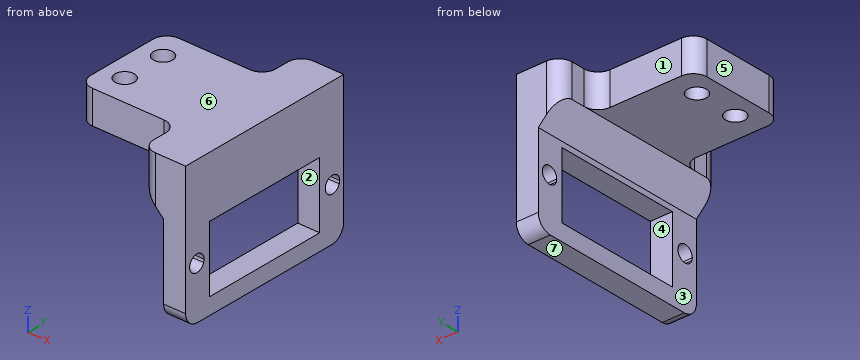
```python
from build123d import *

# Parameters (mm, degrees)
F0_W      = 4
F0_H      = 18
F1_DEPTH  = 26
F0_W_2    = 7
F2_DEPTH  = 6
F3_W      = 4
F3_H      = 18
F4_DEPTH  = 15
F5_W      = 4
F5_H      = 18
F6_DEPTH  = 15
F7_W      = 11.5
F7_H      = 5.5
F7_H_2    = 6
F7_H_3    = 0.5
F8_DEPTH  = 25
F9_DEPTH  = 15
F10_DEPTH = 18
F11_DEPTH = 2
F12_DEPTH = 6
F13_DEPTH = 6
F14_DEPTH = 11
F15_W     = 9
F15_H     = 8
F16_DEPTH = 30
F18_D     = 3.5
F19_W     = 18
F19_H     = 6
F20_DEPTH = 9
F21_W     = 18
F21_H     = 6
F22_DEPTH = 9
F23_SIZE  = 4
F24_DEPTH = 1.5
F25_DEPTH = 1.5
F26_R     = 2.5


with BuildPart() as f1:
    # F0 (on Top) → F1 (new body)
    with BuildSketch(Plane.XY):
        with Locations((9, 9)):
            Rectangle(F0_W, F0_H)
    extrude(amount=-F1_DEPTH)

    # F0 (on Top) → F2 (join)
    with BuildSketch(Plane.XY):
        with Locations((3.5, 9)):
            Rectangle(F0_W_2, F0_H)
        with Locations((9, 9)):
            Rectangle(F0_W, F0_H)
    extrude(amount=-F2_DEPTH)

    # F3 (on face) → F4 (join)
    with BuildSketch(Plane.XZ):
        with Locations((9, -17)):
            Rectangle(F3_W, F3_H)
    extrude(amount=F4_DEPTH)

    # F5 (on face) → F6 (join)
    with BuildSketch(Plane(origin=(0, 18, 0), x_dir=(-1, 0, 0), z_dir=(0, 1, 0))):
        with Locations((-9, -17)):
            Rectangle(F5_W, F5_H)
    extrude(amount=F6_DEPTH)

    # F7 (on face) → F8 (cut)
    with BuildSketch(Plane.YZ.offset(11)):
        with Locations((3.25, -13.75)):
            Rectangle(F7_W, F7_H)
        with Locations((14.75, -13.75)):
            Rectangle(F7_W, F7_H)
        with BuildLine():
            Line((24.5675133947, -17), (21.7390862699, -17))
            ThreePointArc((21.7390862699, -17), (23.1532998323, -18), (24.5675133947, -17))
        make_face()
        with BuildLine():
            Line((24.6532998323, -16.5), (21.6532998323, -16.5))
            ThreePointArc((21.6532998323, -16.5), (21.6749019928, -16.7536529681), (21.7390862699, -17))
            Line((21.7390862699, -17), (24.5675133947, -17))
            ThreePointArc((24.5675133947, -17), (24.6316976718, -16.7536529681), (24.6532998323, -16.5))
        make_face()
        with BuildLine():
            ThreePointArc((24.6532998323, -16.5), (23.1532998323, -15), (21.6532998323, -16.5))
            Line((21.6532998323, -16.5), (24.6532998323, -16.5))
        make_face()
        with Locations((14.75, -20)):
            Rectangle(F7_W, F7_H_2)
        with Locations((14.75, -16.75)):
            Rectangle(F7_W, F7_H_3)
        with Locations((3.25, -20)):
            Rectangle(F7_W, F7_H_2)
        with Locations((3.25, -16.75)):
            Rectangle(F7_W, F7_H_3)
        with BuildLine():
            ThreePointArc((-3.6532998323, -16.5), (-5.1532998323, -15), (-6.6532998323, -16.5))
            Line((-6.6532998323, -16.5), (-3.6532998323, -16.5))
        make_face()
        with BuildLine():
            Line((-3.6532998323, -16.5), (-6.6532998323, -16.5))
            ThreePointArc((-6.6532998323, -16.5), (-6.6316976718, -16.7536529681), (-6.5675133947, -17))
            Line((-6.5675133947, -17), (-3.7390862699, -17))
            ThreePointArc((-3.7390862699, -17), (-3.6749019928, -16.7536529681), (-3.6532998323, -16.5))
        make_face()
        with BuildLine():
            Line((-3.7390862699, -17), (-6.5675133947, -17))
            ThreePointArc((-6.5675133947, -17), (-5.1532998323, -18), (-3.7390862699, -17))
        make_face()
    extrude(amount=-F8_DEPTH, mode=Mode.SUBTRACT)

    # F9 (add): a face of the model
    f9_faces = [f1.faces().sort_by_distance(p)[0] for p in [
        (0, 9, -3),
    ]]
    extrude(f9_faces, amount=F9_DEPTH)

    # F10 (add): a face of the model
    f10_faces = [f1.faces().sort_by_distance(p)[0] for p in [
        (-1.4634146341, 0, -3.1951219512),
    ]]
    extrude(f10_faces, amount=F10_DEPTH)

    # F11 (cut): a face of the model
    f11_faces = [f1.faces().sort_by_distance(p)[0] for p in [
        (-1.4634146341, 18, -3.1951219512),
    ]]
    extrude(f11_faces, amount=-F11_DEPTH, mode=Mode.SUBTRACT)

    # F12 (cut): a face of the model
    f12_faces = [f1.faces().sort_by_distance(p)[0] for p in [
        (9, -15, -17),
    ]]
    extrude(f12_faces, amount=-F12_DEPTH, mode=Mode.SUBTRACT)

    # F13 (cut): a face of the model
    f13_faces = [f1.faces().sort_by_distance(p)[0] for p in [
        (9, 33, -17),
    ]]
    extrude(f13_faces, amount=-F13_DEPTH, mode=Mode.SUBTRACT)

    # F14 (add): a face of the model
    f14_faces = [f1.faces().sort_by_distance(p)[0] for p in [
        (-1.4634146341, 16, -3.1951219512),
    ]]
    extrude(f14_faces, amount=F14_DEPTH)

    # F15 (on face) → F16 (cut)
    with BuildSketch(Plane.YZ.offset(11)):
        with Locations((-13.5, -4)):
            Rectangle(F15_W, F15_H)
    extrude(amount=-F16_DEPTH, mode=Mode.SUBTRACT)

    # F18 (through all)
    with Locations(Plane.XY):
        with Locations((-11, 13), (-11, 5)):
            Hole(F18_D / 2)

    # F19 (on face) → F20 (cut)
    with BuildSketch(Plane.XZ.offset(9)):
        with Locations((-6, -3)):
            Rectangle(F19_W, F19_H)
    extrude(amount=-F20_DEPTH, mode=Mode.SUBTRACT)

    # F21 (on face) → F22 (cut)
    with BuildSketch(Plane(origin=(0, 27, 0), x_dir=(-1, 0, 0), z_dir=(0, 1, 0))):
        with Locations((6, -3)):
            Rectangle(F21_W, F21_H)
    extrude(amount=-F22_DEPTH, mode=Mode.SUBTRACT)

    # F23
    f23_edges = [f1.edges().sort_by_distance(p)[0] for p in [
        (7, 9, -6),
    ]]
    chamfer(f23_edges, length=F23_SIZE)

    # F24 (cut): a face of the model
    f24_faces = [f1.faces().sort_by_distance(p)[0] for p in [
        (8.0980392157, -9, -10.9019607843),
    ]]
    extrude(f24_faces, amount=-F24_DEPTH, mode=Mode.SUBTRACT)

    # F25 (cut): a face of the model
    f25_faces = [f1.faces().sort_by_distance(p)[0] for p in [
        (8.0980392157, 27, -10.9019607843),
    ]]
    extrude(f25_faces, amount=-F25_DEPTH, mode=Mode.SUBTRACT)

    # F26
    f26_edges = [f1.edges().sort_by_distance(p)[0] for p in [
        (9, 25.5, -26),
        (3, 25.5, -3),
        (-15, 18, -3),
        (9, -7.5, -26),
        (3, -7.5, -3),
        (3, 0, -3),
        (3, 18, -3),
        (-15, 0, -3),
    ]]
    fillet(f26_edges, radius=F26_R)


solid = f1.part
```
Can you work these out from the model? Positions are in its coordinate system, mm. Face numbers are marked on the shaded views. A direction names the side the tool comes from. Round coordinates to 2 decimals unless told otherwise and drop trailing zeros. Order: outer loops, then holes, each group sorted by start corner. A loop starts at its lowest first (then second) coordinate and runs counter-clockwise, first axis right, second up. Notation, with made-up numbers: (-19, 88) -> (-5, 88) arc R20 cw to (-5, 110) -> close; hole circle Ø4 at (87.5, 24.25). An arc over 180 degrees is marked (long way). Return JSON: item names as keys, results as strings. Group by question number.
1. If we section it at C-C, the plane z = -22.5: Write out the boundary of the cut face in (x, y), then the cut area to 3 significant figures.
2. If we section it at B-B, the plane y = -1: Write out the boundary of the cut face in (x, z).
3. I need wall thicknesses on line 1 (Y direction, x = -11, z = -3.75); line 2 (Y direction, x = -9.75, z = -1.25); line 3 (Y direction, x = 7.5, z = -12.25). Which ranges of each line are inside material? Lowest first, please. Write a range as [from, to].
4. We'd pull the mould along Z, two halves only. Please class the marked faces 4, 5, 6 and 7: released by +Z, released by -Z, zero draft, split by the parting line, or undercut.
5. Will these pins go through, and if not, where does the flat tip stop? pin 1 (1.5 mm diameter, centred on x = -8.5, y = 20, fed in from +Z); pin 2 (5 mm diameter, centred on x = -7, z = -3.5, fed in from +Y); pin 3 (1 mm diameter, centred on x = 3, y = 21, fed in from -Z); pin 4 (1.8 mm diameter, centred on x = -3, z = -4, fed in from -Y).
6. Which directions (+Z, -Z, +X, -X, +Y, -Y) give clear straight access to the entire face, cutting with the end or side of a thin tool? Please do the marked faces 1, 2 and 3.
7. If we section it at A-A, the plane x = -11: Write out the boundary of the cut face in (y, z), then the cut area to 3 significant figures.
8. If we section it at D-D, the plane y = 13: Write out the boundary of the cut face in (x, z).
Output values:
{
 "1": {"outline": "(7, -7.5) -> (11, -7.5) -> (11, -2.5) -> (7, -2.5) -> close; (7, 20.5) -> (11, 20.5) -> (11, 25.5) -> (7, 25.5) -> close", "area": "40.0 mm²"},
 "2": {"outline": "(2.5, -6) -> (3, -6) -> (7, -10) -> (7, -11) -> (11, -11) -> (11, 0) -> (2.5, 0) -> close; (7, -26) -> (11, -26) -> (11, -23) -> (7, -23) -> close"},
 "3": {"line 1": "[0, 3.25], [6.75, 11.25], [14.75, 18]", "line 2": "[0, 3.78], [6.22, 11.78], [14.22, 18]", "line 3": "[-7.5, -2.5], [20.5, 25.5]"},
 "4": {"face 4": "undercut", "face 5": "zero draft", "face 6": "released by +Z", "face 7": "released by -Z"},
 "5": {"pin 1": "through", "pin 2": "y = 18", "pin 3": "z = -6.5", "pin 4": "y = 0"},
 "6": {"face 1": "+Z, -Z, -X, +Y", "face 2": "+X, -X", "face 3": "-Z, -X, +Y, -Y"},
 "7": {"outline": "(0, -6) -> (3.25, -6) -> (3.25, 0) -> (0, 0) -> close; (6.75, -6) -> (11.25, -6) -> (11.25, 0) -> (6.75, 0) -> close; (14.75, -6) -> (18, -6) -> (18, 0) -> (14.75, 0) -> close", "area": "66.0 mm²"},
 "8": {"outline": "(-15, -6) -> (-12.75, -6) -> (-12.75, 0) -> (-15, 0) -> close; (-9.25, -6) -> (3, -6) -> (7, -10) -> (7, -11) -> (11, -11) -> (11, 0) -> (-9.25, 0) -> close; (7, -26) -> (11, -26) -> (11, -23) -> (7, -23) -> close"}
}
